from build123d import *

# Parameters (mm, degrees)
SKETCH_1_R                  = 200
SKETCH_1_R_2                = 195
EXTRUDE_339_DEPTH           = 500
CUT_EXTRUDE_START           = -127.878338
SKETCH_8_W                  = 244
SKETCH_8_H                  = 41.8
CUT_EXTRUDE_600_DEPTH       = 47.878338
SKETCH_9_R                  = 36
CUT_EXTRUDE_1494_DEPTH      = 575.456264654
CUT_EXTRUDE_1675_REACH      = 576.456
CUT_EXTRUDE_1675_END_RADIUS = 200
SKETCH_10_R                 = 36
SKETCH_14_W                 = 24.14269203
SKETCH_14_H                 = 10
CUT_REVOLVE_1_ANGLE         = 8.5
CUT_EXTRUDE_1_REACH         = 559.136
PATTERN_CIRCULAR_1_COUNT    = 4


with BuildPart() as part:
    # 草图1 → Extrude 339 (new body)
    with BuildSketch(Plane(origin=(0, 0, 0), x_dir=(1, 0, 0), z_dir=(0, 1, 0))):
        with Locations(Location((0, 0, 0), (0, 0, 270))):
            Circle(SKETCH_1_R)
        with Locations(Location((0, 0, 0), (0, 0, 270))):
            Circle(SKETCH_1_R_2, mode=Mode.SUBTRACT)
    extrude(amount=EXTRUDE_339_DEPTH)

    # 草图8 → Cut-Extrude 600 (cut)
    with BuildSketch(Plane.XY.offset(280).offset(CUT_EXTRUDE_START)):
        with Locations((0, 20.9)):
            Rectangle(SKETCH_8_W, SKETCH_8_H)
    extrude(amount=CUT_EXTRUDE_600_DEPTH, mode=Mode.SUBTRACT)

    # 草图9 → Cut-Extrude 1494 (cut, through all)
    with BuildSketch(Plane(origin=(0, 0, 0), x_dir=(0, 0, -1), z_dir=(1, 0, 0))):
        with Locations((0, 180)):
            Circle(SKETCH_9_R)
    extrude(amount=-CUT_EXTRUDE_1494_DEPTH, mode=Mode.SUBTRACT)

    # Cut-Extrude 1675: up to this cylinder (the profile starts inside it)
    cut_extrude_1675_end = Plane(origin=(0, 320, 0), z_dir=(0, -1, 0)) * Cylinder(CUT_EXTRUDE_1675_END_RADIUS, 1553.912, mode=Mode.PRIVATE)
    # 草图10 → Cut-Extrude 1675 (cut, up to the surface)
    with BuildSketch(Plane(origin=(0, 0, 0), x_dir=(0, 0, -1), z_dir=(1, 0, 0)), mode=Mode.PRIVATE) as cut_extrude_1675_sk1:
        with Locations((0, 320)):
            Circle(SKETCH_10_R)
    cut_extrude_1675_tool1 = extrude(cut_extrude_1675_sk1.sketch, amount=-CUT_EXTRUDE_1675_REACH, mode=Mode.PRIVATE) & cut_extrude_1675_end
    add(cut_extrude_1675_tool1.solids().sort_by_distance((0, 320, 0))[0], mode=Mode.SUBTRACT)

    # 草图14 → 切除-旋转1 (revolve, cut)
    with BuildSketch(Plane(origin=(0, 0, 0), x_dir=(0.7313537016191752, 0, 0.6819983600624934), z_dir=(-0.6819983600624934, 0, 0.7313537016191752))):
        with Locations((-187.928653985, 475)):
            Rectangle(SKETCH_14_W, SKETCH_14_H)
    cut_revolve_1 = revolve(axis=Axis((0, -25.014655285, 0), (0, -1, 0)), revolution_arc=CUT_REVOLVE_1_ANGLE, mode=Mode.SUBTRACT)

    # 草图16 → 切除-拉伸1 (cut, up to next)
    with BuildSketch(Plane.XZ.offset(-480), mode=Mode.PRIVATE) as cut_extrude_1_sk1:
        with BuildLine():
            Line((-124.502927328, -156.52163137), (-121.390354144, -152.608590586))
            ThreePointArc((-121.390354144, -152.608590586), (-127.28815173, -147.725171955), (-132.989680212, -142.613971816))
            Line((-132.989680212, -142.613971816), (-136.399672013, -146.270740324))
            ThreePointArc((-136.399672013, -146.270740324), (-130.551950493, -151.512996877), (-124.502927328, -156.52163137))
        make_face()
    cut_extrude_1_tool1 = extrude(cut_extrude_1_sk1.sketch, amount=-CUT_EXTRUDE_1_REACH, mode=Mode.PRIVATE) & part.part
    cut_extrude_1 = cut_extrude_1_tool1.solids().sort_by_distance((-128.893802, 480, -149.588621))[0]
    add(cut_extrude_1, mode=Mode.SUBTRACT)

    # 阵列(圆周)1: 切除-旋转1, 切除-拉伸1 ×4 about axis
    pattern_circular_1_axis = Axis((0, -25.014655285, 0), (0, 1, 0))
    add([cut_revolve_1.rotate(pattern_circular_1_axis, i * 360 / PATTERN_CIRCULAR_1_COUNT) for i in range(1, PATTERN_CIRCULAR_1_COUNT)], mode=Mode.SUBTRACT)
    add([cut_extrude_1.rotate(pattern_circular_1_axis, i * 360 / PATTERN_CIRCULAR_1_COUNT) for i in range(1, PATTERN_CIRCULAR_1_COUNT)], mode=Mode.SUBTRACT)


solid = part.part
For this review, take the finished solid that the model builds, in its own axes (mm). A direction names the side the tool comes from. Round coordinates to 2 decimals unless told otherwise and drop trailing zeros. Write each loop counter-clockwise with the first axis right and the second up, starting at its lowest first coordinate (ties: lowest second). Pieces come first, ordered by that corner, then holes. Notation, with made-up numbers: (87.25, 8.25) - (108.25, 8.25) arc R32 cw to (108.25, 42.25) - close; hole circle Ø10 at (-26, 73.25). An arc over 180 degrees is marked (long way). Use a Markdown table: item, result.
Q1. We need section A-A (x = 0). Give the boundary of the cut face in (y, z), plus the area to 3 significant figures.
Derived:
| item | result |
|---|---|
| outline | (0, -200) - (500, -200) - (500, -195) - (0, -195) - close; (41.8, 195) - (500, 195) - (500, 200) - (41.8, 200) - close |
| area | 4,790 mm2 |
Q2. Machinability: for faces 1 (the flat face through (140, 480, -139)), 2 (the flat face through (-139, 480, -140)), 3 (the cylindrical face through (-195.768, 321.583, 35.965)), which of the approach directions +Z, -Z, +X, -X, +Y, -Y give a long, thin tool a straight path to every point of the face, cutting with its end or side? Answer none if there is none.
Derived:
| item | result |
|---|---|
| face 1 | +X |
| face 2 | -Z |
| face 3 | -X |
Q3. We need section C-C (z = 114.5). Give the boundary of the cut face in (x, y), plus the area to 3 significant figures.
Derived:
| item | result |
|---|---|
| outline | (-163.98, 0) - (-157.84, 0) - (-157.84, 500) - (-163.98, 500) - close; (157.84, 0) - (163.98, 0) - (163.98, 500) - (157.84, 500) - close |
| area | 6,140 mm2 |
Q4. The part is to be moulded in two halves that separate along Y. For faces 4 (the flat face through (22, 500, -194)), 5 (the flat face through (145, 470, -134)), 6 (the flat face through (75, 0, -181)), say which applies: pulls with the +Y half, pulls with the -Y half, needs draft (parallel to the pull), parting line crosses it, or undercut.
Derived:
| item | result |
|---|---|
| face 4 | pulls with the +Y half |
| face 5 | undercut |
| face 6 | pulls with the -Y half |
Q5. We need section B-B (z = 0). Give the boundary of the cut face in (x, y), plus the area to 3 significant figures.
Derived:
| item | result |
|---|---|
| outline | (-200, 0) - (-195, 0) - (-195, 144) - (-200, 144) - close; (-200, 216) - (-195, 216) - (-195, 284) - (-200, 284) - close; (-200, 356) - (-195, 356) - (-195, 500) - (-200, 500) - close; (195, 0) - (200, 0) - (200, 500) - (195, 500) - close |
| area | 4,280 mm2 |
Q6. We need section D-D (y = 380). Give the boundary of the cut face in (x, z), plus the area to 3 significant figures.
Derived:
| item | result |
|---|---|
| outline | circle Ø400 at (0, 0); hole circle Ø390 at (0, 0) |
| area | 6,200 mm2 |
Q7. Wall thickness on line 1 along Y through (x, z) = (-198, 0); line 2 along X through (y, z) = (117.5, 0): over which ranges is each line inside the solid? List them lowest first.
Derived:
| item | result |
|---|---|
| line 1 | y = 0 to 144, 216 to 284, 356 to 500 |
| line 2 | x = -200 to -195, 195 to 200 |
Q8. Clearance check with flat-ended pins moving along their axes: pin 1 (1 mm diameter, centred on x = -19.5, y = 108, fed in from +Z); pin 2 (6 mm diameter, centred on x = 139.5, y = 73.5, fed in from -Z); pin 3 (2 mm diameter, centred on x = -104.5, y = 430.5, fed in from +Z). State where each tip first meets the part, or that it passes through.
Derived:
| item | result |
|---|---|
| pin 1 | stops at z = 199.1 |
| pin 2 | stops at z = -146.18 |
| pin 3 | stops at z = 171.14 |
